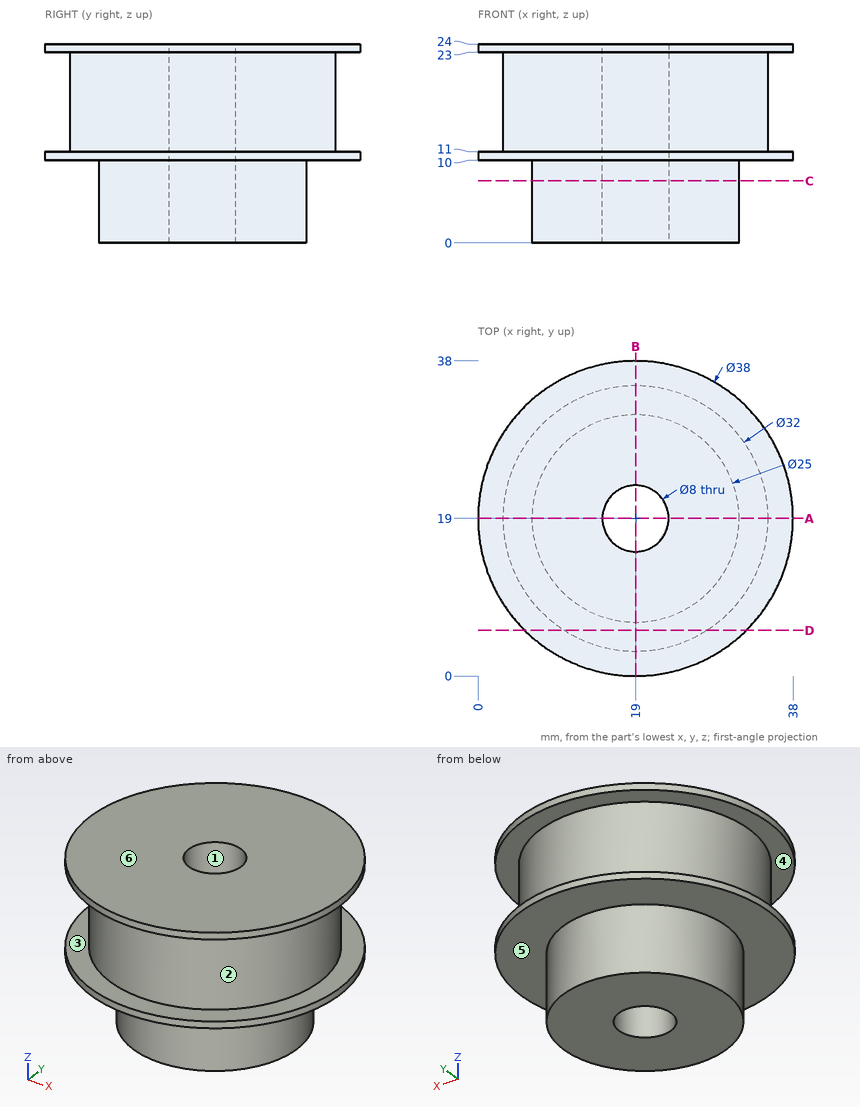
Drawing for the job (mm, zero at the part's lowest x, y, z). A direction names the side the tool comes from. Round coordinates to 2 decimals unless told otherwise and drop trailing zeros. Loops run counter-clockwise (first coordinate to the right, second up) from the corner with the lowest first, then second, coordinate; pieces in that order, holes last.
1. Band-saw the part on C-C, the plane z = 7.5. List the corners of the cut face in (x, y), and give its area (3 significant figures).
Check values:
outline: circle Ø25 at (19, 19); hole circle Ø8 at (19, 19)
area: 441 mm2
2. Drop flat-ended pins along their axis: P1, Ø11.5, axis at x = 15.5, y = 26.5, coming from the -Z side; P2, Ø1, axis at y = 30.5, z = 17.5, coming from the -X side; P3, Ø5, axis at x = 9, z = 17, coming from the -Y side; P4, Ø5, axis at x = 19, y = 19, coming from the -Z side. Give the stop position or say it passes through.
Check values:
P1: stops at z = 0
P2: stops at x = 7.38
P3: stops at y = 4.87
P4: passes through
3. Band-saw the part on D-D, the plane y = 5.5. List the corners of the cut face in (x, z).
Check values:
outline: (5.63, 10) - (32.37, 10) - (32.37, 11) - (27.59, 11) - (27.59, 23) - (32.37, 23) - (32.37, 24) - (5.63, 24) - (5.63, 23) - (10.41, 23) - (10.41, 11) - (5.63, 11) - close
4. Band-saw the part on A-A, the plane y = 19. List the corners of the cut face in (x, z).
Check values:
outline: (0, 10) - (6.5, 10) - (6.5, 0) - (15, 0) - (15, 24) - (0, 24) - (0, 23) - (3, 23) - (3, 11) - (0, 11) - close; (23, 0) - (31.5, 0) - (31.5, 10) - (38, 10) - (38, 11) - (35, 11) - (35, 23) - (38, 23) - (38, 24) - (23, 24) - close
5. Tool access for the marked faces 4, 5 and 6: list every direction of +Z, -Z, +X, -X, +Y, -Y with a clear straight run to the whole face (end or side of a thin tool).
Check values:
face 4: none
face 5: -Z
face 6: +Z, +X, -X, +Y, -Y
6. Mould opens along Y. For the marked faces 1, 2 and 3 say: +Y half, -Y half, draft (parallel to the pull), parting line (faces both ways), or undercut.
Check values:
face 1: undercut
face 2: parting line
face 3: draft
7. Wall check: probe 1 along Y at (x, z) = (19, 13.25); probe 2 along Y at (x, z) = (19, 8.75); probe 3 along Z at (x, y) = (34.5, 10). Give the ranges that are in metal, low to high.
Check values:
probe 1: y = 3 to 15, 23 to 35
probe 2: y = 6.5 to 15, 23 to 31.5
probe 3: z = 10 to 11, 23 to 24
